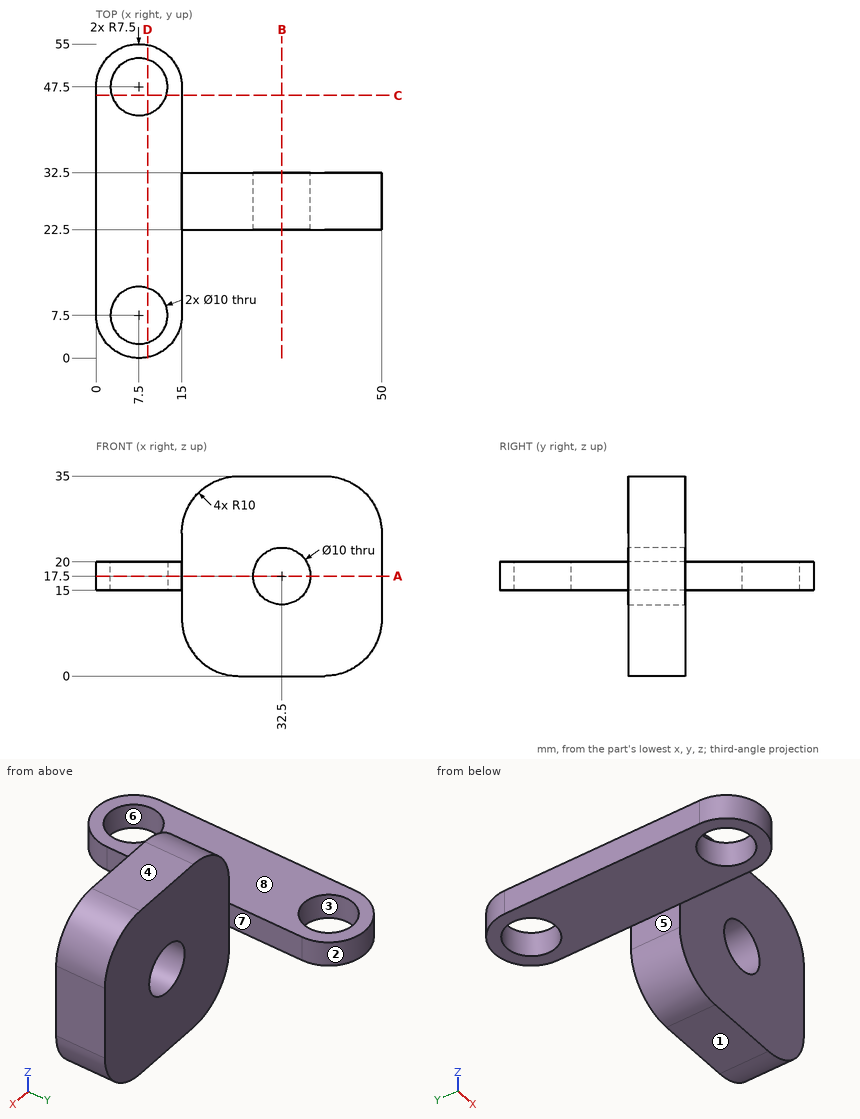
Can you work these out from the drawing? Everything is in mm from the part's minimum corner. A direction names the side the tool comes from. Round coordinates to 2 decimals unless told otherwise and drop trailing zeros. Order: outer loops, then holes, each group sorted by start corner. A loop starts at its lowest first (then second) coordinate and runs counter-clockwise, first axis right, second up. Notation, with made-up numbers: (39, 31) -> (94, 31) arc R28 ccw to (94, 52) -> close; hole circle Ø2 at (21, -13). An arc over 180 degrees is marked (long way). Return JSON: item names as keys, results as strings. Group by question number.
1. If we section it at A-A, the plane z = 17.5: Write out the boundary of the cut face in (x, y), then the cut area to 3 significant figures.
2. We'd pull the mould along X, two halves only. Please class the marked faces 1, 2 and 3: released by +X, released by -X, zero draft, split by the parting line, or undercut.
3. If we section it at C-C, the plane y = 46: Write out the boundary of the cut face in (x, z).
4. Will these pins go through, and if not, where does the flat tip stop? pin 1 (11.5 mm diameter, centred on x = 7.5, y = 47.5, fed in from +Z); pin 2 (6 mm diameter, centred on x = 32, z = 13.5, fed in from -Y); pin 3 (2 mm diameter, centred on x = 36, z = 20, fed in from +Y); pin 4 (6 mm diameter, centred on x = 7.5, y = 7.5, fed in from -Z).
5. If we section it at D-D, the plane x = 9: Write out the boundary of the cut face in (y, z), then the cut area to 3 significant figures.
6. I need wall thicknesses on line 1 (Y direction, x = 7.5, z = 16.1); line 2 (X direction, y = 28, z = 17.5); line 3 (Y direction, x = 19, z = 4). Which ranges of each line are inside material? Lowest first, please. Write a range as [from, to].
7. If we section it at B-B, the plane x = 32.5: Write out the boundary of the cut face in (y, z), then the cut area to 3 significant figures.
8. Which directions (+Z, -Z, +X, -X, +Y, -Y) give clear straight access to the entire face, cutting with the end or side of a thin tool? Please do the marked faces 4, 5, 6, 7 and 8.
Output values:
{
 "1": {"outline": "(0, 7.5) arc R7.5 ccw to (15, 7.5) -> (15, 22.5) -> (27.5, 22.5) -> (27.5, 32.5) -> (15, 32.5) -> (15, 47.5) arc R7.5 ccw to (0, 47.5) -> close; (37.5, 22.5) -> (50, 22.5) -> (50, 32.5) -> (37.5, 32.5) -> close; hole circle Ø10 at (7.5, 7.5); hole circle Ø10 at (7.5, 47.5)", "area": "870 mm²"},
 "2": {"face 1": "zero draft", "face 2": "split by the parting line", "face 3": "undercut"},
 "3": {"outline": "(0, 15) -> (2.73, 15) -> (2.73, 20) -> (0, 20) -> close; (12.27, 15) -> (15, 15) -> (15, 20) -> (12.27, 20) -> close"},
 "4": {"pin 1": "z = 20", "pin 2": "y = 22.5", "pin 3": "y = 32.5", "pin 4": "through"},
 "5": {"outline": "(0.15, 15) -> (2.73, 15) -> (2.73, 20) -> (0.15, 20) -> close; (12.27, 15) -> (42.73, 15) -> (42.73, 20) -> (12.27, 20) -> close; (52.27, 15) -> (54.85, 15) -> (54.85, 20) -> (52.27, 20) -> close", "area": "178 mm²"},
 "6": {"line 1": "[0, 2.5], [12.5, 42.5], [52.5, 55]", "line 2": "[0, 27.5], [37.5, 50]", "line 3": "[22.5, 32.5]"},
 "7": {"outline": "(22.5, 0) -> (32.5, 0) -> (32.5, 12.5) -> (22.5, 12.5) -> close; (22.5, 22.5) -> (32.5, 22.5) -> (32.5, 35) -> (22.5, 35) -> close", "area": "250 mm²"},
 "8": {"face 4": "+Z, +X, -X, +Y, -Y", "face 5": "-Z, -X, +Y, -Y", "face 6": "+Z, -Z", "face 7": "+Z, -Z, +X, +Y", "face 8": "+Z, -X, +Y, -Y"}
}
